Source: three-view drawing plus pictorial views. Frame: mm from the lowest corner of the part. Give positions to 0.01 mm unless a question says otherwise; leave off trailing zeros. Order: outer loops, then holes, each group sorted by start corner. A loop starts at its lowest first (then second) coordinate and runs counter-clockwise, first axis right, second up.
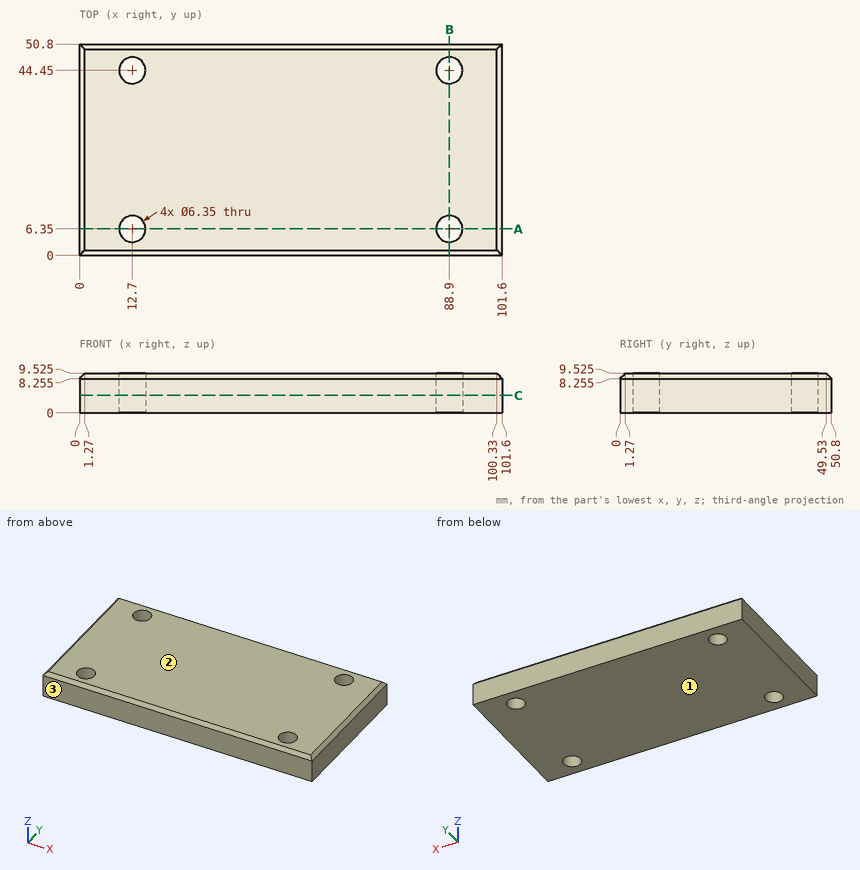
1) Pull-direction query (Z, two-part tool) for the marked faces 1, 2 and 3; classes: +Z half, -Z half, draft (parallel to the pull), parting line (faces both ways), or undercut.
Checks:
face 1: -Z half
face 2: +Z half
face 3: draft
2) Ray query, L1, parallel to Y at x = 12.7, z = 6.75 (3 decimals); L2, parallel to X at y = 6, z = 8; L3, parallel to X at y = 7.5, z = 3. Return the intervals inside material, ascending.
Checks:
L1: y = 0 to 3.175, 9.525 to 41.275, 47.625 to 50.8
L2: x = 0 to 9.54, 15.86 to 85.74, 92.06 to 101.6
L3: x = 0 to 9.74, 15.66 to 85.94, 91.86 to 101.6
3) Section query A-A on y = 6.35. Output: boundary loops of the cut face in (x, z) (3 decimals).
Checks:
outline: (0, 0) - (9.525, 0) - (9.525, 9.525) - (1.27, 9.525) - (0, 8.255) - close; (15.875, 0) - (85.725, 0) - (85.725, 9.525) - (15.875, 9.525) - close; (92.075, 0) - (101.6, 0) - (101.6, 8.255) - (100.33, 9.525) - (92.075, 9.525) - close
4) Section query C-C on z = 4.25. Output: boundary loops of the cut face in (x, y) (3 decimals), and give its area (3 significant figures).
Checks:
outline: (0, 0) - (101.6, 0) - (101.6, 50.8) - (0, 50.8) - close; hole circle Ø6.35 at (12.7, 6.35); hole circle Ø6.35 at (12.7, 44.45); hole circle Ø6.35 at (88.9, 6.35); hole circle Ø6.35 at (88.9, 44.45)
area: 5,030 mm2
5) Section query B-B on x = 88.9. Output: boundary loops of the cut face in (y, z) (3 decimals), and give its area (3 significant figures).
Checks:
outline: (0, 0) - (3.175, 0) - (3.175, 9.525) - (1.27, 9.525) - (0, 8.255) - close; (9.525, 0) - (41.275, 0) - (41.275, 9.525) - (9.525, 9.525) - close; (47.625, 0) - (50.8, 0) - (50.8, 8.255) - (49.53, 9.525) - (47.625, 9.525) - close
area: 361 mm2
